Here's the drawing with two shaded views (mm, measured from the low corner). I have some questions. Give positions to 0.01 mm unless a question says otherwise; leave off trailing zeros. Loops run counter-clockwise (first coordinate to the right, second up) from the corner with the lowest first, then second, coordinate; pieces in that order, holes last. Notation, with made-up numbers: M -34.5,8 L -16.5,8 A22 ccw -16.5,30 Z; hole C 83,-40 d1. An arc over 180 degrees is marked long. Answer in a Markdown table with one row per item. Add a question column.
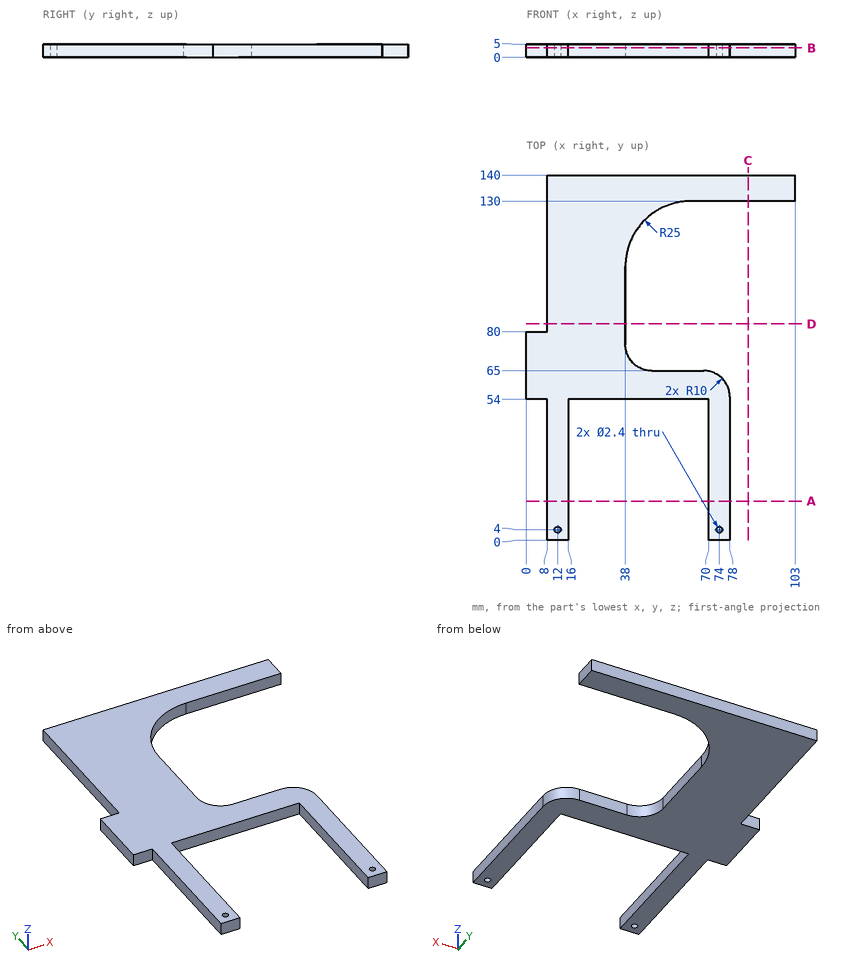
Item 1: Suppose I cut it at D-D (y = 83). List the corners of the cut face in (x, z) for me.
Item 2: I need wall thicknesses on L1, parallel to Y at x = 74, z = 1.35; L2, parallel to X at y = 37, z = 0.9; L3, parallel to X at y = 133, z = 4.5. Which ranges of each line are inside material? Lowest first, please.
Item 3: Suppose I cut it at A-A (y = 15). List the corners of the cut face in (x, z) for me.
Item 4: For P1, Ø2.5, axis at x = 54.5, z = 2.5, coming from the -Y side; P2, Ø1.5, axis at y = 22.5, z = 3.5, coming from the +X side; P3, Ø1.5, axis at y = 100, z = 2.5, coming from the -X side, each with a flat end and sliding along its axis, tell me the tip position at first contact or that it passes through.
Item 5: Suppose I cut it at B-B (z = 3.55). List the corners of the cut face in (x, y) for me.
Item 6: Suppose I cut it at C-C (x = 85). List the corners of the cut face in (y, z) for me.
Values found:
| question | item | result |
|---|---|---|
| 1 | outline | M 8,0 L 38,0 L 38,5 L 8,5 Z |
| 2 | L1 | 0 to 2.8, 5.2 to 63, 130 to 140 |
| 2 | L2 | 8 to 16, 70 to 78 |
| 2 | L3 | 8 to 103 |
| 3 | outline | M 8,0 L 16,0 L 16,5 L 8,5 Z; M 70,0 L 78,0 L 78,5 L 70,5 Z |
| 4 | P1 | y = 54 |
| 4 | P2 | x = 78 |
| 4 | P3 | x = 8 |
| 5 | outline | M 0,54 L 8,54 L 8,0 L 16,0 L 16,54 L 70,54 L 70,0 L 78,0 L 78,55 A10 ccw 68,65 L 48,65 A10 cw 38,75 L 38,105 A25 cw 63,130 L 103,130 L 103,140 L 8,140 L 8,80 L 0,80 Z; hole C 12,4 d2.4; hole C 74,4 d2.4 |
| 6 | outline | M 130,0 L 140,0 L 140,5 L 130,5 Z |
